```python
from build123d import *

# Parameters (mm, degrees)
F1_DEPTH = 25
F2_W     = 20
F2_H     = 20
F3_DEPTH = 10
F3_TAPER = 5
F5_DEPTH = 5
F6_R     = 4
F6_R_2   = 2.5
F7_DEPTH = 6
F8_DEPTH = 45
F9_R     = 1
F10_R    = 1
F11_R    = 1


with BuildPart() as f1:
    # F0 (on Front) → F1 (new body, symmetric)
    with BuildSketch(Plane.XZ):
        Polygon((-50, 0), (0, 0), (50, 0), (50, 25), (20, 42.3205080757), (-20, 42.3205080757), (-50, 25), align=None)
    extrude(amount=F1_DEPTH, both=True)

    # F2 (on face) → F3 (join)
    with BuildSketch(Plane.XY.offset(42.3205080757)):
        Rectangle(F2_W, F2_H)
    extrude(amount=F3_DEPTH, taper=F3_TAPER)

    # F4 (on face) → F5 (join)
    with BuildSketch(Plane.XY.offset(52.3205080757)):
        Polygon((6.2786841774, 3.625), (0, 7.25), (-6.2786841774, 3.625), (-6.2786841774, -3.625), (0, -7.25), (6.2786841774, -3.625), align=None)
    extrude(amount=F5_DEPTH)

    # F6 (on face) → F7 (join)
    with BuildSketch(Plane.XY.offset(57.3205080757)):
        Circle(F6_R)
        Circle(F6_R_2, mode=Mode.SUBTRACT)
    extrude(amount=F7_DEPTH)

    # F8 (add): a face of the model
    f8_faces = [f1.faces().sort_by_distance(p)[0] for p in [
        (0, 0, 57.3205080757),
    ]]
    extrude(f8_faces, amount=-F8_DEPTH)

    # F9
    f9_edges = [f1.edges().sort_by_distance(p)[0] for p in [
        (9.125113, 0, 52.320508),
        (0, -9.125113, 52.320508),
        (-9.125113, 0, 52.320508),
        (0, 9.125113, 52.320508),
    ]]
    fillet(f9_edges, radius=F9_R)

    # F10
    f10_edges = [f1.edges().sort_by_distance(p)[0] for p in [
        (-4, 0, 63.320508),
    ]]
    fillet(f10_edges, radius=F10_R)

    # F11
    f11_edges = [f1.edges().sort_by_distance(p)[0] for p in [
        (-20, 0, 42.320508),
        (20, 0, 42.320508),
        (50, 0, 25),
        (-50, 0, 25),
    ]]
    fillet(f11_edges, radius=F11_R)


solid = f1.part
```
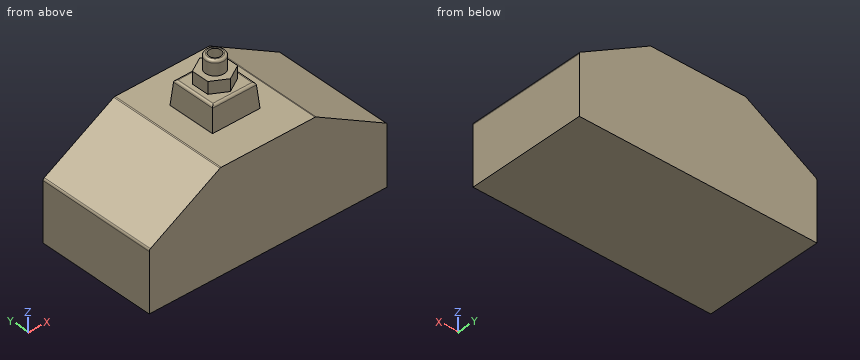
Could you check a few things on this model? Use its own coordinates, in mm. Round coordinates to 2 decimals unless told otherwise and drop trailing zeros. Write each loop counter-clockwise with the first axis right and the second up, starting at its lowest first coordinate (ties: lowest second). Pieces come first, ordered by that corner, then holes. Notation, with made-up numbers: M -35,34 L 19,34 A34 ccw 19,67 Z; hole C -14.75,-5 d11. An arc over 180 degrees is marked long. Answer in a Markdown table with one row per item. Add a question column.
Q1. Imagine slicing it at D-D (z = 39.5). Please give me the cut outline in (x, y), then the cut area to 3 significant figures.
Q2. Will these pins go through, and if not, where does the flat tip stop? pin 1 Ø1.5 at (y, z) = (1.5, 54.5) entering from -X; pin 2 Ø2.5 at (y, z) = (-1.5, 54) entering from +X; pin 3 Ø5 at (y, z) = (2, 45) entering from +X.
Q3. Imagine slicing it at A-A (y = -11.5). Please give me the cut outline in (x, z), then the cut area to 3 significant figures.
Q4. If I drill on line 1 (Y direction, x = 0, z = 60.85); line 2 (Z direction, x = 7.5, y = -18); line 3 (Z direction, x = 7, y = -1.5), over which ranges is the centre line in solid material (lowest first)? Write a range as from..to.
Q5. Imagine slicing it at B-B (x = 12.5). Please give me the cut outline in (y, z).
Values:
| question | item | result |
|---|---|---|
| 1 | outline | M -24.89,-25 L 24.89,-25 L 24.89,25 L -24.89,25 Z |
| 1 | area | 2,490 mm^2 |
| 2 | pin 1 | x = -6.28 |
| 2 | pin 2 | x = 6.28 |
| 2 | pin 3 | x = 9.98 |
| 3 | outline | M -50,0 L 50,0 L 50,24.42 A1 ccw 49.5,25.29 L 20.23,42.19 A1 ccw 19.73,42.32 L -19.73,42.32 A1 ccw -20.23,42.19 L -49.5,25.29 A1 ccw -50,24.42 Z |
| 3 | area | 3,710 mm^2 |
| 4 | line 1 | -4..-2.5, 2.5..4 |
| 4 | line 2 | 0..42.32 |
| 4 | line 3 | 0..52.32 |
| 5 | outline | M -25,0 L 25,0 L 25,42.32 L -25,42.32 Z |
